Check sheet for the modelled part. Datum: model origin and axes. Units: mm. Coordinates: 2 decimals unless noted, no trailing zeros. Order: outer loops, then holes, each group sorted by start corner. A loop starts at its lowest first (then second) coordinate and runs counter-clockwise, first axis right, second up. Notation, with made-up numbers: (-38, -5.5) -> (-7, -5.5) arc R21 cw to (-7, 11.5) -> close; hole circle Ø11 at (-16.5, -31.5). An arc over 180 degrees is marked (long way). Put each result on its own line as item: value. Start each with the question number.
```python
from build123d import *

# Parameters (mm, degrees)
BOSS_EXTRUDE1_DEPTH   = 6.35
CUT_EXTRUDE1_DEPTH    = 6.35
M4_CLEARANCE_HOLE1_D  = 4.5
F_6_CLEARANCE_HOLE1_D = 3.7973
F_6_CLEARANCE_HOLE2_D = 3.7973


with BuildPart() as part:
    # Sketch1 → Boss-Extrude1 (new body)
    with BuildSketch(Plane(origin=(0, 0, 0), x_dir=(1, 0, 0), z_dir=(0, 1, 0))):
        with BuildLine():
            Line((-34.13125, -148.43125), (34.13125, -148.43125))
            ThreePointArc((34.13125, -148.43125), (114.95355509, -114.95355509), (148.43125, -34.13125))
            Line((148.43125, -34.13125), (148.43125, 34.13125))
            ThreePointArc((148.43125, 34.13125), (114.95355509, 114.95355509), (34.13125, 148.43125))
            Line((34.13125, 148.43125), (-34.13125, 148.43125))
            ThreePointArc((-34.13125, 148.43125), (-114.95355509, 114.95355509), (-148.43125, 34.13125))
            Line((-148.43125, 34.13125), (-148.43125, -34.13125))
            ThreePointArc((-148.43125, -34.13125), (-114.95355509, -114.95355509), (-34.13125, -148.43125))
        make_face()
    extrude(amount=BOSS_EXTRUDE1_DEPTH)

    # Sketch4 → Cut-Extrude1 (cut)
    with BuildSketch(Plane(origin=(0, 6.35, 0), x_dir=(1, 0, 0), z_dir=(0, 1, 0))):
        with BuildLine():
            ThreePointArc((-39.448, 145.804481937), (-49.893930566, 144.330021666), (-59.523633513, 140.021852723))
            ThreePointArc((-59.523633513, 140.021852723), (-63.8175, 132.253581937), (-59.523633513, 124.485311151))
            ThreePointArc((-59.523633513, 124.485311151), (-49.893930566, 120.177142208), (-39.448, 118.702681937))
            Line((-39.448, 118.702681937), (39.448, 118.702681937))
            ThreePointArc((39.448, 118.702681937), (49.893930566, 120.177142208), (59.523633513, 124.485311151))
            ThreePointArc((59.523633513, 124.485311151), (63.8175, 132.253581937), (59.523633513, 140.021852723))
            ThreePointArc((59.523633513, 140.021852723), (49.893930566, 144.330021666), (39.448, 145.804481937))
            Line((39.448, 145.804481937), (-39.448, 145.804481937))
        make_face()
        with BuildLine():
            ThreePointArc((39.448, 120.290181937), (49.454528647, 121.702619905), (58.679163809, 125.829568258))
            ThreePointArc((58.679163809, 125.829568258), (62.23, 132.253581937), (58.679163809, 138.677595616))
            ThreePointArc((58.679163809, 138.677595616), (49.454528647, 142.804543969), (39.448, 144.216981937))
            Line((39.448, 144.216981937), (-39.448, 144.216981937))
            ThreePointArc((-39.448, 144.216981937), (-49.454528647, 142.804543969), (-58.679163809, 138.677595616))
            ThreePointArc((-58.679163809, 138.677595616), (-62.23, 132.253581937), (-58.679163809, 125.829568258))
            ThreePointArc((-58.679163809, 125.829568258), (-49.454528647, 121.702619905), (-39.448, 120.290181937))
            Line((-39.448, 120.290181937), (39.448, 120.290181937))
        make_face(mode=Mode.SUBTRACT)
        with BuildLine():
            Line((-39.448, 120.290181937), (39.448, 120.290181937))
            ThreePointArc((39.448, 120.290181937), (49.454528647, 121.702619905), (58.679163809, 125.829568258))
            ThreePointArc((58.679163809, 125.829568258), (62.23, 132.253581937), (58.679163809, 138.677595616))
            ThreePointArc((58.679163809, 138.677595616), (49.454528647, 142.804543969), (39.448, 144.216981937))
            Line((39.448, 144.216981937), (-39.448, 144.216981937))
            ThreePointArc((-39.448, 144.216981937), (-49.454528647, 142.804543969), (-58.679163809, 138.677595616))
            ThreePointArc((-58.679163809, 138.677595616), (-62.23, 132.253581937), (-58.679163809, 125.829568258))
            ThreePointArc((-58.679163809, 125.829568258), (-49.454528647, 121.702619905), (-39.448, 120.290181937))
        make_face()
        with BuildLine():
            ThreePointArc((-59.523633513, -124.485311151), (-63.8175, -132.253581937), (-59.523633513, -140.021852723))
            ThreePointArc((-59.523633513, -140.021852723), (-49.893930566, -144.330021666), (-39.448, -145.804481937))
            Line((-39.448, -145.804481937), (39.448, -145.804481937))
            ThreePointArc((39.448, -145.804481937), (49.893930566, -144.330021666), (59.523633513, -140.021852723))
            ThreePointArc((59.523633513, -140.021852723), (63.8175, -132.253581937), (59.523633513, -124.485311151))
            ThreePointArc((59.523633513, -124.485311151), (49.893930566, -120.177142208), (39.448, -118.702681937))
            Line((39.448, -118.702681937), (-39.448, -118.702681937))
            ThreePointArc((-39.448, -118.702681937), (-49.893930566, -120.177142208), (-59.523633513, -124.485311151))
        make_face()
        with BuildLine():
            ThreePointArc((-58.679163809, -138.677595616), (-49.454528647, -142.804543969), (-39.448, -144.216981937))
            Line((-39.448, -144.216981937), (39.448, -144.216981937))
            ThreePointArc((39.448, -144.216981937), (49.454528647, -142.804543969), (58.679163809, -138.677595616))
            ThreePointArc((58.679163809, -138.677595616), (62.23, -132.253581937), (58.679163809, -125.829568258))
            ThreePointArc((58.679163809, -125.829568258), (49.454528647, -121.702619905), (39.448, -120.290181937))
            Line((39.448, -120.290181937), (-39.448, -120.290181937))
            ThreePointArc((-39.448, -120.290181937), (-49.454528647, -121.702619905), (-58.679163809, -125.829568258))
            ThreePointArc((-58.679163809, -125.829568258), (-62.23, -132.253581937), (-58.679163809, -138.677595616))
        make_face(mode=Mode.SUBTRACT)
        with BuildLine():
            ThreePointArc((-58.679163809, -125.829568258), (-62.23, -132.253581937), (-58.679163809, -138.677595616))
            ThreePointArc((-58.679163809, -138.677595616), (-49.454528647, -142.804543969), (-39.448, -144.216981937))
            Line((-39.448, -144.216981937), (39.448, -144.216981937))
            ThreePointArc((39.448, -144.216981937), (49.454528647, -142.804543969), (58.679163809, -138.677595616))
            ThreePointArc((58.679163809, -138.677595616), (62.23, -132.253581937), (58.679163809, -125.829568258))
            ThreePointArc((58.679163809, -125.829568258), (49.454528647, -121.702619905), (39.448, -120.290181937))
            Line((39.448, -120.290181937), (-39.448, -120.290181937))
            ThreePointArc((-39.448, -120.290181937), (-49.454528647, -121.702619905), (-58.679163809, -125.829568258))
        make_face()
    extrude(amount=-CUT_EXTRUDE1_DEPTH, mode=Mode.SUBTRACT)

    # M4 Clearance Hole1 (through all)
    with Locations(Plane(origin=(0, 6.35, 0), x_dir=(1, 0, 0), z_dir=(0, 1, 0))):
        with Locations((-16, -103.6875), (16, -103.6875), (22, -60.325), (-10, -60.325), (-10, 60.325), (22, 60.325), (16, 103.6875), (-16, 103.6875)):
            Hole(M4_CLEARANCE_HOLE1_D / 2)

    # #6 Clearance Hole1 (through all)
    with Locations(Plane(origin=(0, 6.35, 0), x_dir=(1, 0, 0), z_dir=(0, 1, 0))):
        with Locations((-101.6, -101.6), (-101.6, 101.6), (101.6, 101.6), (101.6, -101.6), (-127, -76.2), (-127, -50.8), (-127, 50.8), (-127, 76.2), (-101.6, 76.2), (-101.6, 50.8), (-101.6, 25.4), (-101.6, 0), (-101.6, -25.4), (-101.6, -50.8), (-101.6, -76.2), (-76.2, -101.6), (-50.8, -101.6), (-50.8, -76.2), (-76.2, -76.2), (-76.2, -50.8), (-50.8, -50.8), (-50.8, -25.4), (-76.2, -25.4), (-76.2, 0), (-50.8, 0), (-50.8, 25.4), (-76.2, 25.4), (-76.2, 50.8), (-50.8, 50.8), (-50.8, 76.2), (-76.2, 76.2), (-76.2, 101.6), (-50.8, 101.6), (50.8, -101.6), (76.2, -101.6), (101.6, -76.2), (127, -76.2), (127, -50.8), (101.6, -25.4), (101.6, -50.8), (76.2, -25.4), (76.2, -50.8), (76.2, -76.2), (50.8, -76.2), (50.8, -50.8), (50.8, -25.4), (50.8, 0), (76.2, 0), (101.6, 0), (101.6, 25.4), (101.6, 50.8), (101.6, 76.2), (127, 50.8), (127, 76.2), (76.2, 101.6), (50.8, 101.6), (50.8, 76.2), (76.2, 76.2), (76.2, 50.8), (76.2, 25.4), (50.8, 25.4), (50.8, 50.8), (0, 0), (-25.4, -25.4), (-25.4, 0), (-25.4, 25.4), (0, 25.4), (25.4, 25.4), (25.4, 0), (25.4, -25.4), (0, -25.4), (127, -25.4), (127, 0), (127, 25.4), (-127, -25.4), (-127, 0), (-127, 25.4)):
            Hole(F_6_CLEARANCE_HOLE1_D / 2)

    # #6 Clearance Hole2 (through all)
    with Locations(Plane(origin=(0, 6.35, 0), x_dir=(1, 0, 0), z_dir=(0, 1, 0))):
        with Locations((-76.2, -127), (76.2, -127), (76.2, 127), (-76.2, 127)):
            Hole(F_6_CLEARANCE_HOLE2_D / 2)


solid = part.part
```
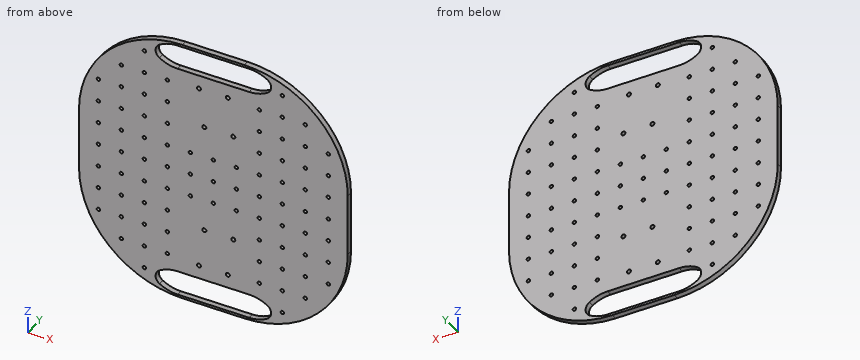
1) Scan lines: line 1 along Z through (x, y) = (25.4, 2); line 2 along Z through (x, y) = (33.5, 4); line 3 along Z through (x, y) = (55.5, 2.75). Record each from-to range of solid material in increasing order. Write a range as [from, to].
2) Sectioned sample at D-D (x = 114). Record the boundary of the cut face in (y, z), plus the area to 3 significant figures.
3) Sectioned sample at C-C (z = -111.5). Record the boundary of the cut face in (x, y).
4) Sectioned sample at B-B (y = 2). State how many separate pieces and enclosed holes the cut face has, plus the area to 3 significant figures.
5) Gauge pin test, flat ends, axial feed: pin 1 (1.5 mm diameter, centred on x = -111.5, y = 4.5, fed in from -Z); pin 2 (3 mm diameter, centred on y = 0.5, z = -75.5, fed in from -X); pin 3 (2 mm diameter, centred on x = 58.5, y = 3, fed in from +Z). Record the tip position at first contact, or that the pin passes through.
6) Sectioned sample at A-A (x = -43.5). Record the boundary of the cut face in (y, z), plus the area to 3 significant figures.
Entries:
1. line 1: z = [-148.43, -145.8], [-118.7, -27.3], [-23.5, -1.9], [1.9, 23.5], [27.3, 118.7], [145.8, 148.43]
1. line 2: z = [-148.43, -145.8], [-118.7, 118.7], [145.8, 148.43]
1. line 3: z = [-146.42, -142.22], [-122.29, 122.29], [142.22, 146.42]
2. outline: (0, -115.9) -> (6.35, -115.9) -> (6.35, 115.9) -> (0, 115.9) -> close
2. area: 1,470 mm2
3. outline: (-118.27, 0) -> (118.27, 0) -> (118.27, 6.35) -> (-118.27, 6.35) -> close
4. separate pieces: 1
4. enclosed holes: 91
4. area: 69,500 mm2
5. pin 1: stops at z = -118.95
5. pin 2: stops at x = -141.25
5. pin 3: stops at z = 146.02
6. outline: (0, -148.05) -> (6.35, -148.05) -> (6.35, -145.59) -> (0, -145.59) -> close; (0, -118.92) -> (6.35, -118.92) -> (6.35, 118.92) -> (0, 118.92) -> close; (0, 145.59) -> (6.35, 145.59) -> (6.35, 148.05) -> (0, 148.05) -> close
6. area: 1,540 mm2
